Could you check a few things on this model? Use its own coordinates, in mm. Face numbers are marked on the shaded views. A direction names the side the tool comes from. Give positions to 0.01 mm unless a question says otherwise; leave off trailing zeros. Loops run counter-clockwise (first coordinate to the right, second up) from the corner with the lowest first, then second, coordinate; pieces in that order, holes last. Notation, with made-up numbers: M 77,56.25 L 105,56.25 A4 cw 105,63.25 Z; hole C 70,85.25 d8. An arc over 180 degrees is marked long. Use a Markdown table: item, result. Add a question column.
1) If I drill on line 1 along Y through (x, z) = (15, 46.05); line 2 along X through (y, z) = (29, 48); line 3 along Y through (x, z) = (8, 42), over which ranges is the centre line in solid material (lowest first)? Write a range as [from, to].
2) Suppose I cut it at A-A on y = 29. List the corners of the cut face in (x, z) for me, and give its area (3 significant figures).
3) Suppose I cut it at D-D on x = 37.5. List the corners of the cut face in (y, z) for me, and give its area (3 significant figures).
4) Which directions (+Z, -Z, +X, -X, +Y, -Y) give clear straight access to the entire face, cutting with the end or side of a thin tool? Please do the marked faces 4 and 5.
5) We'd pull the mould along Y, two halves only. Please class the marked faces 1, 2 and 3: +Y half, -Y half, draft (parallel to the pull), parting line (faces both ways), or undercut.
6) Suppose I cut it at C-C on y = 39. List the corners of the cut face in (x, z) for me.
7) Suppose I cut it at B-B on x = 56. List the corners of the cut face in (y, z) for me.
8) Will these pins go through, and if not, where does the flat tip stop? pin 1 Ø19 at (x, y) = (53, 29) entering from +Z; pin 2 Ø11.5 at (x, y) = (15, 29) entering from +Z; pin 3 Ø6 at (x, y) = (15, 45.5) entering from -Z.
```python
from build123d import *

# Parameters (mm, degrees)
SKETCH_W        = 84
SKETCH_H        = 58
SKETCH_R        = 1.5
SKETCH_R_2      = 12
SKETCH_R_3      = 2.5
SKETCH_R_4      = 5
PAD_DEPTH       = 50
SKETCH001_W     = 79
SKETCH001_H     = 48
POCKET_DEPTH    = 45
POCKET001_DEPTH = 58.001
SKETCH003_R     = 3
POCKET002_DEPTH = 84.001
CHAMFER_SIZE    = 4
CHAMFER001_SIZE = 4
CHAMFER002_SIZE = 2
CHAMFER003_SIZE = 2


with BuildPart() as part:
    # Sketch → Pad (new body)
    with BuildSketch(Plane.XY):
        with Locations((42, 29)):
            Rectangle(SKETCH_W, SKETCH_H)
        with Locations((37.5, 44.5)):
            Circle(SKETCH_R, mode=Mode.SUBTRACT)
        with Locations((68.5, 44.5)):
            Circle(SKETCH_R, mode=Mode.SUBTRACT)
        with Locations((68.5, 13.5)):
            Circle(SKETCH_R, mode=Mode.SUBTRACT)
        with Locations((37.5, 13.5)):
            Circle(SKETCH_R, mode=Mode.SUBTRACT)
        with Locations((53, 29)):
            Circle(SKETCH_R_2, mode=Mode.SUBTRACT)
        with Locations((15, 45.5)):
            Circle(SKETCH_R_3, mode=Mode.SUBTRACT)
        with Locations((15, 12.5)):
            Circle(SKETCH_R_3, mode=Mode.SUBTRACT)
        with Locations((15, 29)):
            Circle(SKETCH_R_4, mode=Mode.SUBTRACT)
    extrude(amount=PAD_DEPTH)

    # Sketch001 (on Face13 of Pad) → Pocket (cut)
    with BuildSketch(Plane(origin=(0, 0, 0), x_dir=(1, 0, 0), z_dir=(0, 0, -1))):
        with Locations((39.5, -29)):
            Rectangle(SKETCH001_W, SKETCH001_H)
    extrude(amount=-POCKET_DEPTH, mode=Mode.SUBTRACT)

    # Sketch002 (on Face9 of Pocket) → Pocket001 (cut, through all)
    with BuildSketch(Plane.XZ):
        Polygon((0, 45), (0, 0), (79, 0), align=None)
    extrude(amount=-POCKET001_DEPTH, mode=Mode.SUBTRACT)

    # Sketch003 (on Face4 of Pocket001) → Pocket002 (cut, through all)
    with BuildSketch(Plane.YZ.offset(84)):
        with Locations((14.5, 20)):
            Circle(SKETCH003_R)
        with Locations((43.5, 20)):
            Circle(SKETCH003_R)
    extrude(amount=-POCKET002_DEPTH, mode=Mode.SUBTRACT)

    # Chamfer
    chamfer_edges = [part.edges().sort_by_distance(p)[0] for p in [
        (0, 58, 47.5),
        (0, 0, 47.5),
    ]]
    chamfer(chamfer_edges, length=CHAMFER_SIZE)

    # Chamfer001
    chamfer001_edges = [part.edges().sort_by_distance(p)[0] for p in [
        (81.5, 0, 0),
        (81.5, 58, 0),
    ]]
    chamfer(chamfer001_edges, length=CHAMFER001_SIZE)

    # Chamfer002
    chamfer002_edges = [part.edges().sort_by_distance(p)[0] for p in [
        (84, 29, 50),
    ]]
    chamfer(chamfer002_edges, length=CHAMFER002_SIZE)

    # Chamfer003
    chamfer003_edges = [part.edges().sort_by_distance(p)[0] for p in [
        (83, 0, 49),
        (83, 58, 49),
    ]]
    chamfer(chamfer003_edges, length=CHAMFER003_SIZE)


solid = part.part
```
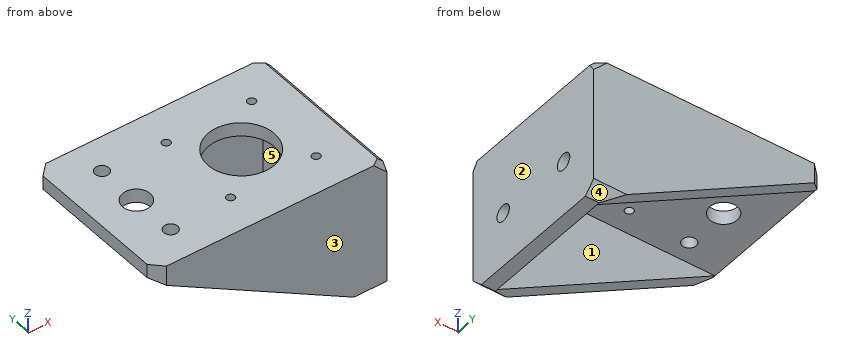
Answer block:
| question | item | result |
|---|---|---|
| 1 | line 1 | y = [0, 10], [15, 24], [34, 43], [48, 58] |
| 1 | line 2 | x = [0, 10], [20, 41], [65, 84] |
| 1 | line 3 | y = [0, 5], [53, 58] |
| 2 | outline | M 0,45 L 10,45 L 10,50 L 0,50 Z; M 20,45 L 41,45 L 41,50 L 20,50 Z; M 65,45 L 79,45 L 79,0 L 84,0 L 84,48 L 82,50 L 65,50 Z |
| 2 | area | 473 mm^2 |
| 3 | outline | M 0,23.64 L 5,23.64 L 5,45 L 12,45 L 12,50 L 0,50 Z; M 15,45 L 43,45 L 43,50 L 15,50 Z; M 46,45 L 53,45 L 53,23.64 L 58,23.64 L 58,50 L 46,50 Z |
| 3 | area | 474 mm^2 |
| 4 | face 4 | -Z, +X, -X, +Y |
| 4 | face 5 | -Z, -X |
| 5 | face 1 | undercut |
| 5 | face 2 | draft |
| 5 | face 3 | -Y half |
| 6 | outline | M 0,45 L 46.37,45 L 46.37,50 L 0,50 Z; M 59.63,45 L 79,45 L 79,0 L 84,0 L 84,48 L 82,50 L 59.63,50 Z |
| 7 | outline | M 0,13.1 L 5,13.1 L 5,45 L 17.38,45 L 17.38,50 L 0,50 Z; M 40.62,45 L 53,45 L 53,13.1 L 58,13.1 L 58,50 L 40.62,50 Z |
| 8 | pin 1 | passes through |
| 8 | pin 2 | stops at z = 50 |
| 8 | pin 3 | stops at z = 45 |
